Can you work these out from the drawing? Everything is in mm from the part's minimum corner. A direction names the side the tool comes from. Round coordinates to 2 decimals unless told otherwise and drop trailing zeros. Write each loop counter-clockwise with the first axis right and the second up, starting at its lowest first coordinate (ties: lowest second). Pieces come first, ordered by that corner, then holes. Notation, with made-up numbers: M -22,18.5 L 4,18.5 A23 ccw 4,41.5 Z; hole C 32.5,27 d8. An arc over 180 degrees is marked long. Answer in a Markdown table with one row per item. Add a question column.
(1) Suppose I cut it at A-A, the plane x = 5.5. Write out the boundary of the cut face in (y, z) (1 decimal), then the cut area to 3 significant figures.
(2) Suppose I cut it at B-B, the plane y = 13. Write out the boundary of the cut face in (x, z) (1 decimal).
(3) If I drill on probe 1 along Y at (x, z) = (3.25, 4.5); probe 2 along Y at (x, z) = (6, 3.75); probe 3 along Z at (x, y) = (3, 3.25) (1 decimal), over which ranges is the centre line in solid material (lowest first)?
(4) If we mould it in two halves opening along X, with no side actions, what happens to the marked faces 1, 2 and 3? For each: released by +X, released by -X, zero draft, split by the parting line, or undercut.
(5) For the marked faces 4 and 5, which set-ups out of +Z, -Z, +X, -X, +Y, -Y let a thin tool reach every point of the face, with its end or its side?
(6) I'm going to push flat-ended pins straight in: pin 1 (4 mm diameter, centred on y = 8, z = 1.5, fed in from -X); pin 2 (4 mm diameter, centred on x = 8, y = 5, fed in from +Z); pin 3 (1 mm diameter, centred on x = 6, y = 6, fed in from +Z). Where does each tip first touch, or does it pass through?
(7) Suppose I cut it at C-C, the plane z = 4.5. Write out the boundary of the cut face in (x, y) (1 decimal).
(8) Suppose I cut it at D-D, the plane y = 2. Write out the boundary of the cut face in (x, z) (1 decimal).
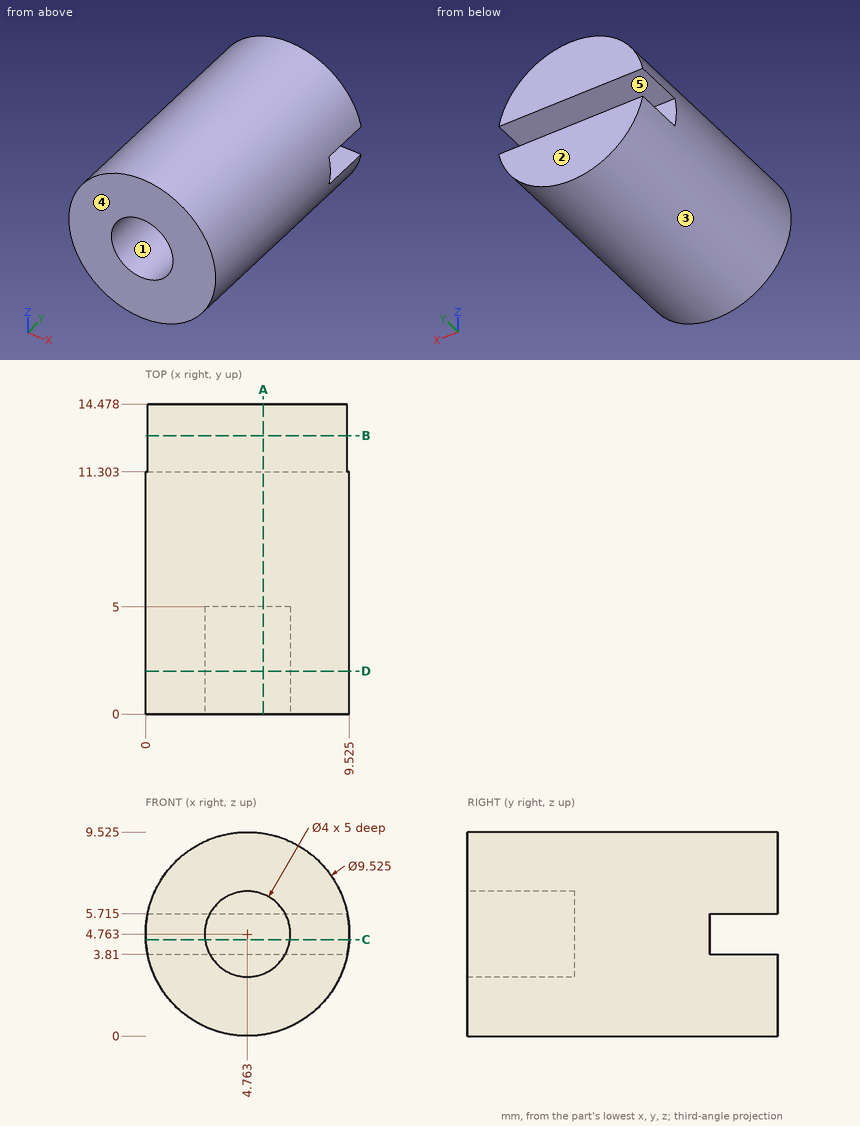
Calculated:
| question | item | result |
|---|---|---|
| 1 | outline | M 0,0.1 L 14.5,0.1 L 14.5,3.8 L 11.3,3.8 L 11.3,5.7 L 14.5,5.7 L 14.5,9.5 L 0,9.5 L 0,6.6 L 5,6.6 L 5,2.9 L 0,2.9 Z |
| 1 | area | 112 mm² |
| 2 | outline | M 0.1,3.8 A4.8 ccw 9.4,3.8 Z; M 0.1,5.7 L 9.4,5.7 A4.8 ccw Z |
| 3 | probe 1 | 5 to 11.3 |
| 3 | probe 2 | 5 to 14.48 |
| 3 | probe 3 | 0.3 to 3.8, 5.7 to 9.2 |
| 4 | face 1 | undercut |
| 4 | face 2 | zero draft |
| 4 | face 3 | split by the parting line |
| 5 | face 4 | +Z, -Z, +X, -X, -Y |
| 5 | face 5 | +X, -X, +Y |
| 6 | pin 1 | x = 0.17 |
| 6 | pin 2 | z = 9.36 |
| 6 | pin 3 | z = 9.47 |
| 7 | outline | M 0,0 L 2.8,0 L 2.8,5 L 6.7,5 L 6.7,0 L 9.5,0 L 9.5,11.3 L 0,11.3 Z |
| 8 | outline | C 4.8,4.8 d9.5; hole C 4.8,4.8 d4 |
